The listing builds one solid part. Answer for the finished solid, in the listing's coordinates (mm). Coordinates: 2 decimals unless noted, no trailing zeros. Loops run counter-clockwise (first coordinate to the right, second up) from the corner with the lowest first, then second, coordinate; pieces in that order, holes last. Notation, with made-up numbers: M 27.25,-2 L 75.25,-2 A25 ccw 75.25,20 Z; hole C 86.5,34.5 d1. An arc over 180 degrees is marked long. Answer as a JSON object with one key per item and string values. Group by question number.
1. A cutting plane is placed at B-B on x = 6. Give the vertices of the cut face in (y, z).
2. A cutting plane is placed at A-A on x = -116.5. Give the vertices of the cut face in (y, z), and give its area (3 significant figures).
3. Given pin 1 (1.5 mm diameter, centred on x = -296.5, z = 3.5, fed in from -Y), flat-ended and moving along its own axis, determine where the tip first touches the part or whether it passes through.
4. Determine the mould class of faces 1 (the face through (-93, 109, 0)), 2 (the face through (80.417, 80.864, 2.535)) for opening direction Y: released by +Y, released by -Y, zero draft, split by the parting line, or undercut.
5. Straight lines are drawn through the part: L1, parallel to Y at x = -151, z = 1.2 (3 decimals); L2, parallel to Y at x = 7, z = 4.25; L3, parallel to Y at x = -61, z = 0.4. For each, find the intervals that lie inside material, in ascending order.
from build123d import *

# Parameters (mm, degrees)
SKETCH1_W           = 180
SKETCH1_H           = 130
BOSS_EXTRUDE1_DEPTH = 5
SKETCH2_W           = 130
SKETCH2_H           = 80
CUT_EXTRUDE1_DEPTH  = 10
SKETCH5_R           = 1.625
BOSS_EXTRUDE3_DEPTH = 5
SKETCH6_W           = 112.5
SKETCH6_H           = 130
BOSS_EXTRUDE4_DEPTH = 5
SKETCH7_W           = 5
SKETCH7_H           = 5
CUT_EXTRUDE2_DEPTH  = 5
BOSS_EXTRUDE5_DEPTH = 5
SKETCH9_R           = 2.5
CUT_EXTRUDE3_DEPTH  = 5
SKETCH10_R          = 16
SKETCH10_W          = 22
SKETCH10_H          = 26
CUT_EXTRUDE4_DEPTH  = 5


with BuildPart() as part:
    # Sketch1 → Boss-Extrude1 (new body)
    with BuildSketch(Plane.XY):
        with Locations((-90, 65)):
            Rectangle(SKETCH1_W, SKETCH1_H)
    extrude(amount=BOSS_EXTRUDE1_DEPTH)

    # Sketch2 → Cut-Extrude1 (cut)
    with BuildSketch(Plane.XY.offset(5)):
        with Locations((-90, 65)):
            Rectangle(SKETCH2_W, SKETCH2_H)
    extrude(amount=-CUT_EXTRUDE1_DEPTH, mode=Mode.SUBTRACT)

    # Sketch5 → Boss-Extrude3 (add)
    # profile 1 of 4: a face of its own
    with BuildSketch(Plane.XY.offset(5)):
        with BuildLine():
            Line((-33, 101), (-33, 105))
            Line((-33, 105), (-25, 105))
            Line((-25, 105), (-25, 97))
            Line((-25, 97), (-29, 97))
            ThreePointArc((-29, 97), (-31.828427125, 98.171572875), (-33, 101))
        make_face()
        with Locations((-29, 101)):
            Circle(SKETCH5_R, mode=Mode.SUBTRACT)
    # profile 2 of 4: a face of its own
    with BuildSketch(Plane.XY.offset(5)):
        with BuildLine():
            Line((-155, 97), (-151, 97))
            ThreePointArc((-151, 97), (-148.171572875, 98.171572875), (-147, 101))
            Line((-147, 101), (-147, 105))
            Line((-147, 105), (-155, 105))
            Line((-155, 105), (-155, 97))
        make_face()
        with Locations(Location((-151, 101, 0), (0, 0, 180))):
            Circle(SKETCH5_R, mode=Mode.SUBTRACT)
    # profile 3 of 4: a face of its own
    with BuildSketch(Plane.XY.offset(5)):
        with BuildLine():
            Line((-25, 33), (-29, 33))
            ThreePointArc((-29, 33), (-31.828427125, 31.828427125), (-33, 29))
            Line((-33, 29), (-33, 25))
            Line((-33, 25), (-25, 25))
            Line((-25, 25), (-25, 33))
        make_face()
        with Locations(Location((-29, 29, 0), (0, 0, 180))):
            Circle(SKETCH5_R, mode=Mode.SUBTRACT)
    # profile 4 of 4: a face of its own
    with BuildSketch(Plane.XY.offset(5)):
        with BuildLine():
            Line((-147, 29), (-147, 25))
            Line((-147, 25), (-155, 25))
            Line((-155, 25), (-155, 33))
            Line((-155, 33), (-151, 33))
            ThreePointArc((-151, 33), (-148.171572875, 31.828427125), (-147, 29))
        make_face()
        with Locations((-151, 29)):
            Circle(SKETCH5_R, mode=Mode.SUBTRACT)
    extrude(amount=-BOSS_EXTRUDE3_DEPTH)

    # Sketch6 → Boss-Extrude4 (add)
    with BuildSketch(Plane.XY.offset(5)):
        with Locations((-236.25, 65)):
            Rectangle(SKETCH6_W, SKETCH6_H)
        with Locations((56.25, 65)):
            Rectangle(SKETCH6_W, SKETCH6_H)
    extrude(amount=-BOSS_EXTRUDE4_DEPTH)

    # Sketch7 → Cut-Extrude2 (cut)
    with BuildSketch(Plane.XY.offset(5)):
        with Locations((-290, 37.5)):
            Rectangle(SKETCH7_W, SKETCH7_H)
        with Locations((-290, 92.5)):
            Rectangle(SKETCH7_W, SKETCH7_H)
        with Locations((110, 92.5)):
            Rectangle(SKETCH7_W, SKETCH7_H)
        with Locations((110, 37.5)):
            Rectangle(SKETCH7_W, SKETCH7_H)
    extrude(amount=-CUT_EXTRUDE2_DEPTH, mode=Mode.SUBTRACT)

    # Sketch8 → Boss-Extrude5 (add)
    with BuildSketch(Plane.XY.offset(5)):
        Polygon((-302.5, 40), (-292.5, 40), (-292.5, 45), (-297.5, 45), (-297.5, 85), (-292.5, 85), (-292.5, 90), (-302.5, 90), align=None)
        Polygon((117.5, 85), (117.5, 45), (112.5, 45), (112.5, 40), (122.5, 40), (122.5, 90), (112.5, 90), (112.5, 85), align=None)
    extrude(amount=-BOSS_EXTRUDE5_DEPTH)

    # Sketch9 → Cut-Extrude3 (cut)
    with BuildSketch(Plane.XY.offset(5)):
        with Locations((-252.5, 65)):
            Circle(SKETCH9_R)
        with Locations((-247.737605985, 81.219224524)):
            Circle(SKETCH9_R)
        with Locations((-234.96245039, 92.288959861)):
            Circle(SKETCH9_R)
        with Locations((-218.230554852, 94.694643256)):
            Circle(SKETCH9_R)
        with Locations((-202.854177982, 87.672487231)):
            Circle(SKETCH9_R)
        with Locations((-193.715210792, 73.451976705)):
            Circle(SKETCH9_R)
        with Locations((-193.715210792, 56.548023295)):
            Circle(SKETCH9_R)
        with Locations((-202.854177982, 42.327512769)):
            Circle(SKETCH9_R)
        with Locations((-218.230554852, 35.305356744)):
            Circle(SKETCH9_R)
        with Locations((-234.96245039, 37.711040139)):
            Circle(SKETCH9_R)
        with Locations((-247.737605985, 48.780775476)):
            Circle(SKETCH9_R)
    extrude(amount=-CUT_EXTRUDE3_DEPTH, mode=Mode.SUBTRACT)

    # Sketch10 → Cut-Extrude4 (cut)
    with BuildSketch(Plane.XY.offset(5)):
        with Locations((82.5, 65)):
            Circle(SKETCH10_R)
        with Locations((6.5, 65)):
            Rectangle(SKETCH10_W, SKETCH10_H)
        with Locations((36.5, 65)):
            Rectangle(SKETCH10_W, SKETCH10_H)
    extrude(amount=-CUT_EXTRUDE4_DEPTH, mode=Mode.SUBTRACT)


solid = part.part
From the geometry:
{
 "1": {"outline": "M 0,0 L 52,0 L 52,5 L 0,5 Z; M 78,0 L 130,0 L 130,5 L 78,5 Z"},
 "2": {"outline": "M 0,0 L 25,0 L 25,5 L 0,5 Z; M 105,0 L 130,0 L 130,5 L 105,5 Z", "area": "250 mm²"},
 "3": {"pin 1": "stops at y = 40"},
 "4": {"face 1": "zero draft", "face 2": "undercut"},
 "5": {"L1": "y = 0 to 27.375, 30.625 to 33, 97 to 99.375, 102.625 to 130", "L2": "y = 0 to 52, 78 to 130", "L3": "y = 0 to 25, 105 to 130"}
}
